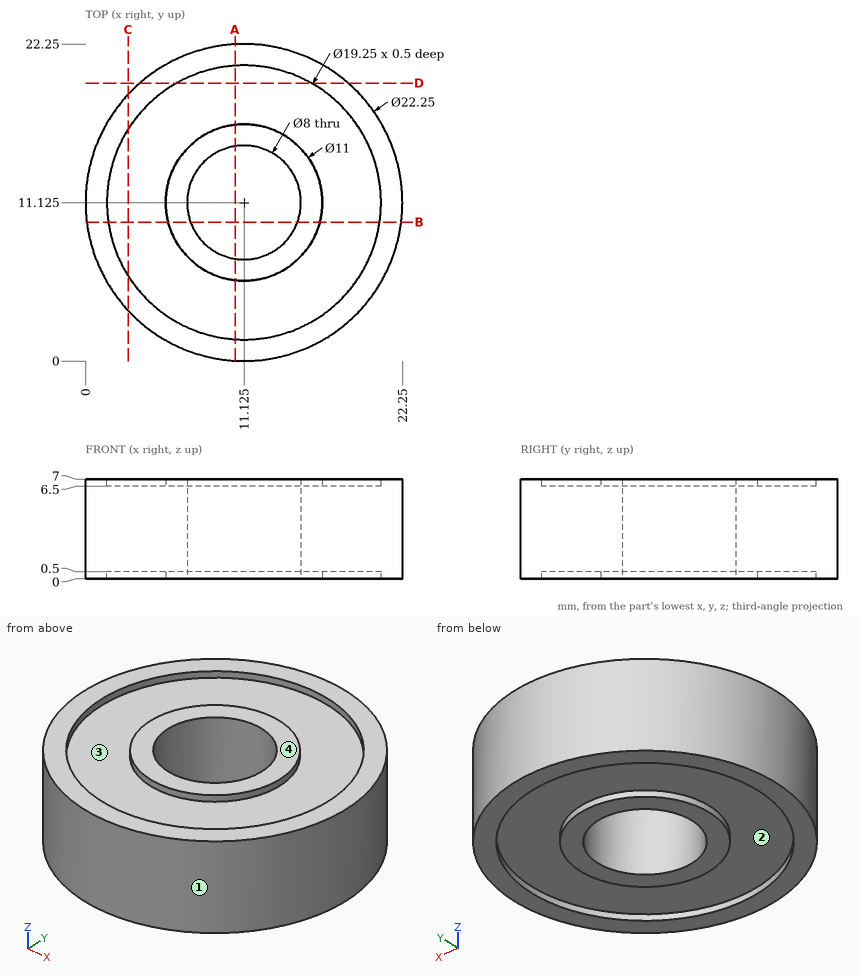
Geometry check sheet. Reference: drawing and pictorial views, mm from the part's lowest x, y, z. Give positions to 0.01 mm unless a question says otherwise; leave off trailing zeros. Order: outer loops, then holes, each group sorted by start corner. A loop starts at its lowest first (then second) coordinate and runs counter-clockwise, first axis right, second up. Notation, with made-up numbers: (65, 29) -> (95, 29) arc R32 cw to (95, 57) -> close; hole circle Ø2 at (41.25, 57.5). An arc over 180 degrees is marked (long way). Write each question's results on one line, items separated by ' | '. Start each with the question number.
(1) Scan lines: line 1 (X direction, y = 11, z = 5.25); line 2 (X direction, y = 8.25, z = 1). Record each from-to range of solid material in increasing order.
(2) Gauge pin test, flat ends, axial feed: P1, Ø1.5, axis at y = 7, z = 5.5, coming from the +X side; P2, Ø3, axis at x = 16, z = 2.5, coming from the -Y side. Record the tip position at first contact, or that the pin passes through.
(3) Sectioned sample at B-B (y = 9.75). Enter the section's corners in (x, z).
(4) Sectioned sample at C-C (x = 3). Enter the section's corners in (y, z).
(5) Sectioned sample at D-D (y = 19.5). Enter the section's corners in (x, z).
(6) Sectioned sample at A-A (x = 10.5). Enter the section's corners in (y, z), plus the area to 3 significant figures.
(7) Mould release check, pull along X, two halves, no side actions. Record for the marked faces 1, 2, 3 and 4: pulls with the +X half, pulls with the -X half, needs draft (parallel to the pull), parting line crosses it, or undercut.
Answer below:
1) line 1: 0 to 7.13, 15.12 to 22.25 | line 2: 0.38 to 8.34, 13.91 to 21.87
2) P1: x = 21.73 | P2: y = 0.52
3) outline: (0.09, 0) -> (1.6, 0) -> (1.6, 0.5) -> (5.8, 0.5) -> (5.8, 0) -> (7.37, 0) -> (7.37, 7) -> (5.8, 7) -> (5.8, 6.5) -> (1.6, 6.5) -> (1.6, 7) -> (0.09, 7) -> close; (14.88, 0) -> (16.45, 0) -> (16.45, 0.5) -> (20.65, 0.5) -> (20.65, 0) -> (22.16, 0) -> (22.16, 7) -> (20.65, 7) -> (20.65, 6.5) -> (16.45, 6.5) -> (16.45, 7) -> (14.88, 7) -> close
4) outline: (3.53, 0) -> (5.97, 0) -> (5.97, 0.5) -> (16.28, 0.5) -> (16.28, 0) -> (18.72, 0) -> (18.72, 7) -> (16.28, 7) -> (16.28, 6.5) -> (5.97, 6.5) -> (5.97, 7) -> (3.53, 7) -> close
5) outline: (3.8, 0) -> (6.38, 0) -> (6.38, 0.5) -> (15.87, 0.5) -> (15.87, 0) -> (18.45, 0) -> (18.45, 7) -> (15.87, 7) -> (15.87, 6.5) -> (6.38, 6.5) -> (6.38, 7) -> (3.8, 7) -> close
6) outline: (0.02, 0) -> (1.52, 0) -> (1.52, 0.5) -> (5.66, 0.5) -> (5.66, 0) -> (7.17, 0) -> (7.17, 7) -> (5.66, 7) -> (5.66, 6.5) -> (1.52, 6.5) -> (1.52, 7) -> (0.02, 7) -> close; (15.08, 0) -> (16.59, 0) -> (16.59, 0.5) -> (20.73, 0.5) -> (20.73, 0) -> (22.23, 0) -> (22.23, 7) -> (20.73, 7) -> (20.73, 6.5) -> (16.59, 6.5) -> (16.59, 7) -> (15.08, 7) -> close | area: 91.9 mm2
7) face 1: parting line crosses it | face 2: undercut | face 3: undercut | face 4: needs draft
